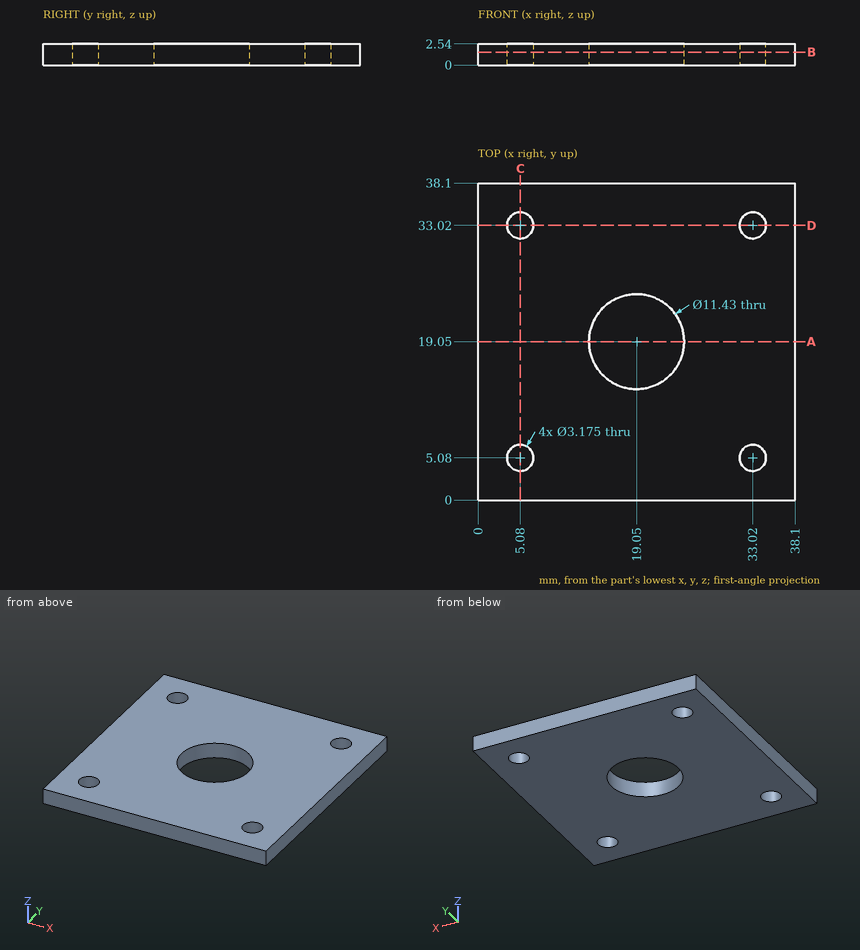
Design review of the part shown in the three views and the two pictorial views. Dimensions are in mm from the part's minimum x, y and z. Round coordinates to 2 decimals unless told otherwise and drop trailing zeros. Order: outer loops, then holes, each group sorted by start corner. A loop starts at its lowest first (then second) coordinate and runs counter-clockwise, first axis right, second up.
Item 1: Add section A-A, the plane y = 19.05. State the section outline as (x, z) points (3 decimals), and give its area (3 significant figures).
Working result:
outline: (0, 0) - (13.335, 0) - (13.335, 2.54) - (0, 2.54) - close; (24.765, 0) - (38.1, 0) - (38.1, 2.54) - (24.765, 2.54) - close
area: 67.7 mm2
Item 2: To check wall thickness, follow probe 1 along X at (y, z) = (33.02, 1.9); probe 2 along Y at (x, z) = (19.05, 1.3) (3 decimals). State the ranges of each line that lie inside material, in increasing order.
Working result:
probe 1: x = 0 to 3.49, 6.67 to 31.43, 34.61 to 38.1
probe 2: y = 0 to 13.335, 24.765 to 38.1
Item 3: Add section C-C, the plane x = 5.08. State the section outline as (y, z) points, and give its area (3 significant figures).
Working result:
outline: (0, 0) - (3.49, 0) - (3.49, 2.54) - (0, 2.54) - close; (6.67, 0) - (31.43, 0) - (31.43, 2.54) - (6.67, 2.54) - close; (34.61, 0) - (38.1, 0) - (38.1, 2.54) - (34.61, 2.54) - close
area: 80.6 mm2
Item 4: For pin 1 (5 mm diameter, centred on x = 20.5, y = 9, fed in from -Z), flat-tipped, find the tip position at first contact; note if it passes through.
Working result:
pin 1: stops at z = 0
Item 5: Add section B-B, the plane z = 1.55. Count the separate pieces of the cut face and the enclosed holes in it, and give its area (3 significant figures).
Working result:
separate pieces: 1
enclosed holes: 5
area: 1,320 mm2
